from build123d import *

# Parameters (mm, degrees)
SZKIC1_W                        = 30
SZKIC1_H                        = 75
DODANIE_WYCI_GNI_CIE1_DEPTH     = 4
DODANIE_WYCI_GNI_CIE9_DEPTH     = 5
ZAOKR_GLENIE4_START             = -20
ZAOKR_GLENIE4_DEPTH             = 6
ZAOKR_GLENIE7_START             = 14
ZAOKR_GLENIE7_DEPTH             = 6
SZKIC12_W                       = 30
SZKIC12_H                       = 85
DODANIE_WYCI_GNI_CIE14_DEPTH    = 7
SZKIC13_W                       = 30
SZKIC13_H                       = 38
WYTNIJ_WYCI_GNI_CIE3_DEPTH      = 10
ZAOKR_GLENIE10_R                = 20
WYTNIJ_WYCI_GNI_CIE4_DEPTH      = 108.491901733
WYTNIJ_WYCI_GNI_CIE4_DEPTH_BACK = 108.491901733
SZKIC16_R                       = 6
ZAOKR_GLENIE11_R                = 10


with BuildPart() as part:
    # Szkic1 → Dodanie-wyciągnięcie1 (new body)
    with BuildSketch(Plane.XY):
        Rectangle(SZKIC1_W, SZKIC1_H)
    extrude(amount=DODANIE_WYCI_GNI_CIE1_DEPTH)

    # Szkic2<6> → Dodanie-wyciągnięcie9 (add)
    with BuildSketch(Plane.ZY.offset(15)):
        with BuildLine():
            Line((-62.531345503, -2.73), (0, -2.73))
            Line((0, -2.73), (0, -37.5))
            Line((0, -37.5), (4, -37.5))
            Line((4, -37.5), (4, -7.5))
            Line((4, -7.5), (89, -7.5))
            Line((89, -7.5), (89, -0.5))
            ThreePointArc((89, -0.5), (36.533874177, 38.142707909), (-27.765672752, 48.703081871))
            Line((-27.765672752, 48.703081871), (-62.531345503, 37.27))
            Line((-62.531345503, 37.27), (-62.531345503, -2.73))
        make_face()
    dodanie_wyci_gni_cie9 = extrude(amount=DODANIE_WYCI_GNI_CIE9_DEPTH)

    # Zaokrąglenie4: read off the stored shape, not the designer's step
    # Zaokrąglenie4 outline → Zaokrąglenie4 (cut)
    with BuildSketch(Plane.YZ.offset(ZAOKR_GLENIE4_START)):
        with BuildLine():
            add(Edge.make_bspline(
                [(46.914284354, -33.205041576), (48.244794, -29.159256091), (48.938225425, -25.023538595), (49.036781903, -20.899990656)],
                knots=[0.800219325, 0.800219325, 0.800219325, 0.800219325, 1, 1, 1, 1], degree=3, weights=[0.909036421, 0.931787704, 0.962108897, 1]))
            Line((46.914284354, -33.205041576), (48.703081871, -27.765672752))
            ThreePointArc((48.703081871, -27.765672752), (48.912277268, -24.334889862), (49.036781903, -20.899990656))
        make_face()
        with BuildLine():
            add(Edge.make_bspline(
                [(6.398511186, -62.531345503), (25.138203193, -62.531345503), (40.842910838, -51.666745261), (46.914284354, -33.205041576)],
                knots=[0, 0, 0, 0, 0.800219325, 0.800219325, 0.800219325, 0.800219325], degree=3, weights=[1, 0.848227597, 0.817906404, 0.909036421]))
            Line((6.398511186, -62.531345503), (37.27, -62.531345503))
            Line((37.27, -62.531345503), (46.914284354, -33.205041576))
        make_face()
    extrude(amount=ZAOKR_GLENIE4_DEPTH, mode=Mode.SUBTRACT)

    # Lustro2: Dodanie-wyciągnięcie9 across plane
    add(dodanie_wyci_gni_cie9.mirror(Plane(origin=(0, 0, 0), x_dir=(0, 0, 1), z_dir=(1, 0, 0))))

    # Zaokrąglenie7: read off the stored shape, not the designer's step
    # Zaokrąglenie7 outline → Zaokrąglenie7 (cut)
    with BuildSketch(Plane.YZ.offset(ZAOKR_GLENIE7_START)):
        with BuildLine():
            ThreePointArc((48.703081871, -27.765672752), (48.912277268, -24.334889862), (49.036781903, -20.899990656))
            add(Edge.make_bspline(
                [(49.036781903, -20.899990656), (48.938225459, -25.023537174), (48.244794476, -29.159253258), (46.914285711, -33.205037449)],
                knots=[0, 0, 0, 0, 0.199780609, 0.199780609, 0.199780609, 0.199780609], degree=3, weights=[1, 0.962108909, 0.931787724, 0.909036443]))
            Line((46.914285711, -33.205037449), (48.703081871, -27.765672752))
        make_face()
        with BuildLine():
            Line((37.27, -62.531345503), (46.914285711, -33.205037449))
            add(Edge.make_bspline(
                [(46.914285711, -33.205037449), (40.842913536, -51.666743395), (25.138205022, -62.531345503), (6.398511186, -62.531345503)],
                knots=[0.199780609, 0.199780609, 0.199780609, 0.199780609, 1, 1, 1, 1], degree=3, weights=[0.909036443, 0.817906399, 0.848227585, 1]))
            Line((6.398511186, -62.531345503), (37.27, -62.531345503))
        make_face()
    extrude(amount=ZAOKR_GLENIE7_DEPTH, mode=Mode.SUBTRACT)

    # Szkic12 → Dodanie-wyciągnięcie14 (add)
    with BuildSketch(Plane.XZ.offset(7.5)):
        with Locations((0, 46.5)):
            Rectangle(SZKIC12_W, SZKIC12_H)
    extrude(amount=-DODANIE_WYCI_GNI_CIE14_DEPTH)

    # Szkic13 → Wytnij-wyciągnięcie3 (cut)
    with BuildSketch(Plane.XY.offset(4)):
        with Locations((0, 18.5)):
            Rectangle(SZKIC13_W, SZKIC13_H)
    extrude(amount=-WYTNIJ_WYCI_GNI_CIE3_DEPTH, mode=Mode.SUBTRACT)

    # Zaokrąglenie10
    zaokr_glenie10_edges = [part.edges().sort_by_distance(p)[0] for p in [
        (17.5, -2.73, -62.531345503),
        (-17.5, -2.73, -62.531345503),
    ]]
    fillet(zaokr_glenie10_edges, radius=ZAOKR_GLENIE10_R)

    # Szkic16 → Wytnij-wyciągnięcie4 (cut, two sides: drawn at the far end of the back side and taken through both)
    with BuildSketch(Plane(origin=(-15, 0, 0), x_dir=(0, 0, -1), z_dir=(1, 0, 0)).offset(-WYTNIJ_WYCI_GNI_CIE4_DEPTH_BACK)):
        with Locations((41.107158155, 15.269526453)):
            Circle(SZKIC16_R)
    extrude(amount=WYTNIJ_WYCI_GNI_CIE4_DEPTH + WYTNIJ_WYCI_GNI_CIE4_DEPTH_BACK, mode=Mode.SUBTRACT)

    # Zaokrąglenie11
    zaokr_glenie11_edges = [part.edges().sort_by_distance(p)[0] for p in [
        (-17.5, -2.73, 0),
        (17.5, -2.73, 0),
    ]]
    fillet(zaokr_glenie11_edges, radius=ZAOKR_GLENIE11_R)


solid = part.part
Geometry: final body of the model. Coordinates: model frame, mm. A direction names the side the tool comes from. Give positions to 0.01 mm unless a question says otherwise; leave off trailing zeros. Loops run counter-clockwise (first coordinate to the right, second up) from the corner with the lowest first, then second, coordinate; pieces in that order, holes last. Notation, with made-up numbers: (-37.5, 18) -> (-21.5, 18) arc R30 ccw to (-21.5, 44) -> close; hole circle Ø5 at (60.25, -12.75). An arc over 180 degrees is marked (long way). Put each result on its own line as item: value.
1. Pull-direction query (X, two-part tool) for faces 1 (the flat face through (17, -2.73, -25)), 2 (the flat face through (-20, 16, 14)), 3 (the flat face through (15, 19, -3)); classes: released by +X, released by -X, zero draft, split by the parting line, or undercut.
Taken from the geometry:
face 1: zero draft
face 2: released by -X
face 3: undercut
2. Cut plane D-D (z = -6). Return the cut outline in (x, y), plus the area to 3 significant figures.
Taken from the geometry:
outline: (-20, -3.56) -> (-15, -3.56) -> (-15, 48.6) -> (-20, 48.6) -> close; (15, -3.56) -> (20, -3.56) -> (20, 48.6) -> (15, 48.6) -> close
area: 522 mm2
3. Set-up query: faces 4 (the flat face through (0, -7.5, 47)), 5 (the flat face through (0, -0.5, 45)), 6 (the flat face through (0, -19, 0)). Return all of +Z, -Z, +X, -X, +Y, -Y with unobstructed straight access to the full face (end or side cutting, diameter ignored); none if empty.
Taken from the geometry:
face 4: +Z, +X, -X, -Y
face 5: +Z, -Z, +Y
face 6: -Z, -Y
4. Cut plane A-A (x = -13.5). Return the cut outline in (y, z), plus the area to 3 significant figures.
Taken from the geometry:
outline: (-37.5, 0) -> (-0.5, 0) -> (-0.5, 89) -> (-7.5, 89) -> (-7.5, 4) -> (-37.5, 4) -> close
area: 743 mm2
5. Ray query, line 1 along X through (y, z) = (40, -33); line 2 along Z through (x, y) = (2, -6.5); line 3 along Z through (x, y) = (0, -12.5). Return the intervals inside material, ascending. Write a range as [from, to].
Taken from the geometry:
line 1: x = [-20, -15], [15, 20]
line 2: z = [0, 89]
line 3: z = [0, 4]
6. Cut plane C-C (y = -30.5). Return the cut outline in (x, z), plus the area to 3 significant figures.
Taken from the geometry:
outline: (-20, 0) -> (20, 0) -> (20, 4) -> (-20, 4) -> close
area: 160 mm2
7. Cut plane B-B (z = 35.5). Return the cut outline in (x, y).
Taken from the geometry:
outline: (-20, -7.5) -> (20, -7.5) -> (20, 38.57) -> (15, 38.57) -> (15, -0.5) -> (-15, -0.5) -> (-15, 38.57) -> (-20, 38.57) -> close
8. Pin query (flat end, axial travel): P1, Ø8, axis at x = 12, y = 10.5, coming from the +Z side; P2, Ø12, axis at x = -13, z = 52.5, coming from the -Y side; P3, Ø18.5, axis at x = 5, y = -24, coming from the -Z side. Return the tip coordinate at first contact, or that it passes through.
Taken from the geometry:
P1: stops at z = 81.36
P2: stops at y = -7.5
P3: stops at z = 0
